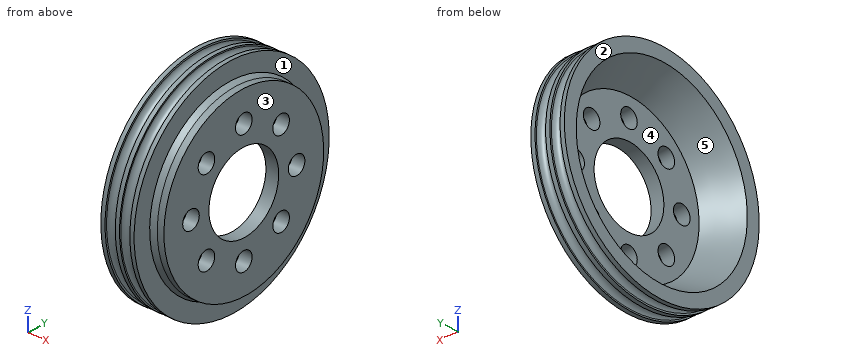
```python
from build123d import *

# Parameters (mm, degrees)
SKETCH2_R          = 4.25
CUT_EXTRUDE1_DEPTH = 10


with BuildPart() as part:
    # Sketch1 → Revolve1 (revolve)
    with BuildSketch(Plane.XY, mode=Mode.PRIVATE) as revolve1_sk:
        with BuildLine():
            Line((1.256075941, 4.83169775), (1.256075941, -3.156564647))
            Line((1.256075941, -3.156564647), (3.835935187, -4.230222841))
            Line((3.835935187, -4.230222841), (6.956075941, -4.230222841))
            Line((6.956075941, -4.230222841), (6.956075941, -27.31830225))
            Line((6.956075941, -27.31830225), (0.956075941, -27.31830225))
            Line((0.956075941, -27.31830225), (0.956075941, -9.230222841))
            Line((0.956075941, -9.230222841), (-14.443924059, -1.328435893))
            Line((-14.443924059, -1.328435893), (-14.443924059, 4.769777159))
            Line((-14.443924059, 4.769777159), (-12.443924059, 4.769777159))
            Line((-12.443924059, 4.769777159), (-12.443924059, 3.983753219))
            ThreePointArc((-12.443924059, 3.983753219), (-10.043924059, 1.583753219), (-7.643924059, 3.983753219))
            Line((-7.643924059, 3.983753219), (-7.643924059, 4.769777159))
            Line((-7.643924059, 4.769777159), (-5.643924059, 4.769777159))
            Line((-5.643924059, 4.769777159), (-5.643924059, 4.15038965))
            ThreePointArc((-5.643924059, 4.15038965), (-3.193924059, 1.70038965), (-0.743924059, 4.15038965))
            Line((-0.743924059, 4.15038965), (-0.743924059, 4.83169775))
            Line((-0.743924059, 4.83169775), (1.256075941, 4.83169775))
        make_face()
    revolve(revolve1_sk.sketch.rotate(Axis((-24.757186567, -45.230222841, 0), (1, 0, 0)), 90), axis=Axis((-24.757186567, -45.230222841, 0), (1, 0, 0)))

    # Sketch2 → Cut-Extrude1 (cut)
    with BuildSketch(Plane.ZY.offset(-0.956075941)):
        with Locations((0, -18.130222841)):
            Circle(SKETCH2_R)
        with Locations((19.16259377, -26.067629071)):
            Circle(SKETCH2_R)
        with Locations((27.1, -45.230222841)):
            Circle(SKETCH2_R)
        with Locations((19.16259377, -64.392816611)):
            Circle(SKETCH2_R)
        with Locations((0, -72.330222841)):
            Circle(SKETCH2_R)
        with Locations((-19.16259377, -64.392816611)):
            Circle(SKETCH2_R)
        with Locations((-27.1, -45.230222841)):
            Circle(SKETCH2_R)
        with Locations((-19.16259377, -26.067629071)):
            Circle(SKETCH2_R)
    extrude(amount=-CUT_EXTRUDE1_DEPTH, mode=Mode.SUBTRACT)


solid = part.part
```
The model under review builds one solid part; all positions refer to its coordinate system, in mm. Face numbers are marked on the shaded views. A direction names the side the tool comes from. Round coordinates to 2 decimals unless told otherwise and drop trailing zeros. Answer as a JSON object with one key per item and string values. Group by question number.
1) Mouldability with a two-part tool opening along Y and no side actions: class the marked faces 3, 4 and 5 as released by +Y, released by -Y, zero draft, split by the parting line, or undercut.
2) For line 1 (Z direction, x = 2.5, y = -43.5); line 2 (X direction, y = -28, z = -44.5); line 3 (X direction, y = -7, z = 30), list the stretches that pass through material, from the lowest coordinate up. Write a range as [from, to].
3) We need section A-A on x = 5. Give the number of separate pieces and of enclosed holes in the cut face, then the cut area to 3 significant figures.
4) For pin 1 Ø6 at (x, y) = (-8, -74.5) entering from +Z; pin 2 Ø13.5 at (y, z) = (-45.23, 27.1) entering from -X; pin 3 Ø8 at (y, z) = (-15, 26.5) entering from -X; pin 4 Ø2 at (x, z) = (-10, -9.5) entering from +Y, all flat-tipped, find the tip position at first contact; note any pin that passes through.
5) For the marked faces 1 and 2, list the 3-axis set-ups (+Z, -Z, +X, -X, +Y, -Y) from which the entire face can be reached by the end or side of a thin tool; tool diameter is ignored.
Result set:
{
 "1": {"face 3": "zero draft", "face 4": "undercut", "face 5": "undercut"},
 "2": {"line 1": "[-41.52, -30.98], [-23.22, -17.83], [17.83, 23.22], [30.98, 41.52]", "line 2": "[-14.44, -11.92], [-8.17, -4.99], [-1.39, 1.26]", "line 3": "[-14.44, -12.36], [-7.72, -5.51], [-0.87, 1.26]"},
 "3": {"separate pieces": "1", "enclosed holes": "9", "area": "3,820 mm²"},
 "4": {"pin 1": "z = 42.53", "pin 2": "x = 0.96", "pin 3": "x = -14.44", "pin 4": "y = 0.9"},
 "5": {"face 1": "+X", "face 2": "+Z, -Z, -X, +Y, -Y"}
}
